Autodesk Inventor part; units mm, degrees
ref_plane "YZ Plane" through (0, 0, 0) normal (1, 0, 0) x (0, 1, 0)
ref_plane "XZ Plane" through (0, 0, 0) normal (0, 1, 0) x (-1, 0, 0)
ref_plane "XY Plane" through (0, 0, 0) normal (0, 0, 1) x (1, 0, 0)
sketch "Sketch1" plane through (0, 0, 0) normal (0, 0, 1) x (1, 0, 0)
  line L0 (0, 0) -> (25.4, 0)
  line L1 (25.4, 0) -> (25.4, 50.8)
  line L2 (25.4, 50.8) -> (0, 50.8)
  line L3 (0, 50.8) -> (0, 0)
  line L4 (1.5875, 1.5875) -> (23.8125, 1.5875)
  line L5 (23.8125, 1.5875) -> (23.8125, 49.2125)
  line L6 (23.8125, 49.2125) -> (1.5875, 49.2125)
  line L7 (1.5875, 49.2125) -> (1.5875, 1.5875)
  dimension "d0" = 25.4
  dimension "d1" = 50.8
  dimension "d2" = 1.5875
extrude "Extrusion1" add sketch "Sketch1" along normal blind 365.252
sketch "Sketch2" plane through (25.4, 0, 0) normal (1, 0, 0) x (0, 0, -1)
  line L0 (0, 50.8) -> (-365.252, 50.8)
  line L1 (-365.252, 50.8) -> (-356.075, 0)
  line L2 (-356.075, 0) -> (-365.252, 0)
  line L3 (0, 1.5875) -> (-365.252, 1.5875)
  line L4 (-365.252, 50.8) -> (-365.252, 0)
  line L5 (-365.252, 0) -> (-365.252, 50.8)
  point P0 (0, 0)
  dimension "d5" = 10.24
sketch "Sketch3" plane through (25.4, 0, 0) normal (1, 0, 0) x (0, 0, -1)
  line L0 (0, 0) -> (0, 50.8)
  line L1 (0, 50.8) -> (-365.252, 50.8)
  line L2 (0, 0) -> (-365.252, 0)
  line L3 (-365.252, 0) -> (-365.252, 50.8)
  point P0 (-50.8, 25.4)
  point P1 (-190.5737, 25.4)
  point P2 (-356.075, 0)
  point P3 (-301.5742, 25.4)
  dimension "d9" = 50.8
  dimension "d10" = 25.4
  dimension "d19" = 25.4
  dimension "d21" = 25.4
  dimension "d25" = 63.6778
  dimension "d28" = 174.6783
hole "Hole1" at (25.4, 25.4, 50.8) at (25.4, 25.4, 190.5737) at (25.4, 25.4, 301.5742) direction (-1, 0, 0) diameter 22.225 depth 25.4 tip angle 118
sketch "Sketch4" plane through (25.4, 0, 0) normal (1, 0, 0) x (0, 0, -1)
  line L0 (0, 50.8) -> (-365.252, 50.8)
  line L1 (-163.5862, 50.8) -> (0, 50.8)
  line L2 (0, 50.8) -> (0, 0)
  line L3 (0, 0) -> (-163.5862, 0)
  line L4 (-163.5862, 0) -> (-163.5862, 50.8)
  circle A0 centre (-190.5737, 25.4) radius 11.1125
  dimension "d22" = 26.9875
extrude "Extrusion3" cut sketch "Sketch4" against normal blind 25.4 contours L2 L3 L4 L0
extrude "Extrusion4" cut sketch "Sketch2" against normal blind 25.4
fillet "Fillet1" radius 12.7 2 edges at (12.7, 50.8, 163.5862) (12.7, 0, 163.5862)
sketch "Sketch5" plane through (25.4, 12.7, 163.5862) normal (1, 0, 0) x (0, 0, -1)
  circle A0 centre (-26.9875, 12.7) radius 11.1125
  circle A1 centre (-137.988, 12.7) radius 11.1125
  point P0 (163.5862, -12.7)
  dimension "d30" = 0
  dimension "d31" = 0
hole "Hole2" at (25.4, 25.4, 190.5737) at (25.4, 25.4, 301.5742) direction (-1, 0, 0) diameter 28.575 depth 1.5875 tip angle 118
properties part number "ARM_030_TopIntakeSide" material "Aluminum 6061"
CAD build for the part. Positions are in the model's coordinates, mm. A direction names the side the tool comes from. Give positions to 0.01 mm unless a question says otherwise; leave off trailing zeros. Order: outer loops, then holes, each group sorted by start corner. A loop starts at its lowest first (then second) coordinate and runs counter-clockwise, first axis right, second up. Notation, with made-up numbers: M -19,37.25 L 1,37.25 A20 cw 1,62.25 Z; hole C -13.5,41 d11. An arc over 180 degrees is marked long. Put each result on its own line as item: value. Start each with the question number.
(1) Which spindle directions (+Z, -Z, +X, -X, +Y, -Y) get a long thin tool onto all of the face, cutting with end or side? Do faces 1 (the cylindrical face through (15.7, 49.55, 170.79)), 2 (the flat face through (23.812, 25, 263)), 3 (the cylindrical face through (24.595, 13.353, 293.893)). Say none if no direction does.
(2) Flat gauge pins, fed straight in: pin 1 Ø1 at (y, z) = (30, 201) entering from +X; pin 2 Ø10 at (x, y) = (3, 11) entering from +Z. Where does each tip first touch, or does it go through?
(3) Drill centre lines: line 1 along Y through (x, z) = (19.75, 312.5); line 2 along X through (y, z) = (37, 228.5); line 3 along Z through (x, y) = (1, 25.4). Where is each one in solid material? Low to high.
(4) Saw through at B-B, the plane z = 337. Write the cut outline in (x, y), then the cut area to 3 significant figures.
(5) Mould opens along Z. For faces 4 (the cylindrical face through (0.783, 24.911, 201.675)), 5 (the flat face through (13, 1.588, 262)), 6 (the cylindrical face through (24.6, 15.74, 201.1)), 7 (the flat face through (0.53, 25.519, 360.685)) say: +Z half, -Z half, draft (parallel to the pull), parting line (faces both ways), or undercut.
(6) Saw through at D-D, the plane y = 25.4. Write the cut outline in (x, z).
(7) Saw through at C-C, the plane y = 44.5. Write the cut outline in (x, z), then the cut area to 3 significant figures.
(8) Saw through at A-A, the plane x = 8.5. Write the cut outline in (y, z) (1 decimal).
Check result:
1. face 1: -Z, +X, -X, +Y
1. face 2: +Z, -Z
1. face 3: +X
2. pin 1: stops at x = 1.59
2. pin 2: stops at z = 358.93
3. line 1: y = 0 to 1.59, 49.21 to 50.8
3. line 2: x = 0 to 1.59, 23.81 to 25.4
3. line 3: z = 163.59 to 179.46, 201.69 to 290.46, 312.69 to 360.66
4. outline: M 0,0 L 25.4,0 L 25.4,50.8 L 0,50.8 Z; hole M 1.59,1.59 L 23.81,1.59 L 23.81,49.21 L 1.59,49.21 Z
4. area: 232 mm2
5. face 4: undercut
5. face 5: draft
5. face 6: undercut
5. face 7: +Z half
6. outline: M 0,163.59 L 1.59,163.59 L 1.59,179.46 L 0,179.46 Z; M 0,201.69 L 1.59,201.69 L 1.59,290.46 L 0,290.46 Z; M 0,312.69 L 1.59,312.69 L 1.59,360.66 L 0,360.66 Z; M 23.81,163.59 L 25.4,163.59 L 25.4,176.29 L 23.81,176.29 Z; M 23.81,204.86 L 25.4,204.86 L 25.4,287.29 L 23.81,287.29 Z; M 23.81,315.86 L 25.4,315.86 L 25.4,360.66 L 23.81,360.66 Z
7. outline: M 0,165.32 L 1.59,165.32 L 1.59,364.11 L 0,364.11 Z; M 23.81,165.32 L 25.4,165.32 L 25.4,364.11 L 23.81,364.11 Z
7. area: 631 mm2
8. outline: M 0,176.3 A12.7 ccw 1.6,170.1 L 1.6,356.4 L 0,356.1 Z; M 49.2,170.1 A12.7 ccw 50.8,176.3 L 50.8,365.3 L 49.2,365 Z
